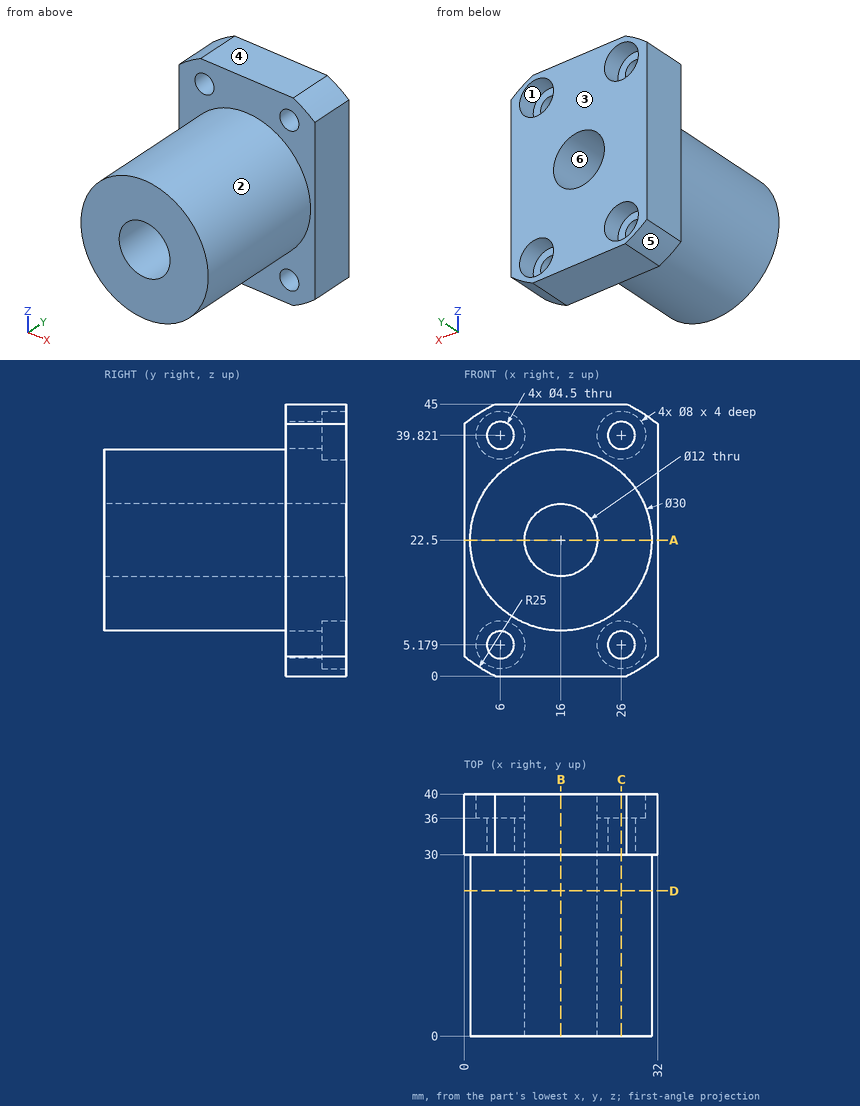
Study the drawing (mm; zero at the part's minimum x, y, z) and answer. A direction names the side the tool comes from. Coordinates: 2 decimals unless noted, no trailing zeros. Write each loop counter-clockwise with the first axis right and the second up, starting at its lowest first coordinate (ties: lowest second). Pieces come first, ordered by that corner, then holes. Notation, with made-up numbers: (29, 68) -> (49, 68) arc R16 cw to (49, 97) -> close; hole circle Ø1 at (61.5, 73.25). An arc over 180 degrees is marked (long way). Write each question's results on one line, items separated by ' | '. Start each with the question number.
1) A tool of negligible diameter and unlimited length cuts with its end or side. For the marked faces 1, 2 and 3, from which of +Z, -Z, +X, -X, +Y, -Y can it reach the whole face along a straight path? Write none if from no direction.
2) Straight lines are drawn through the part: probe 1 along Z at (x, y) = (6, 38.75); probe 2 along Z at (x, y) = (26, 32.8); probe 3 along Y at (x, z) = (25.5, 34.5). For each, find the intervals that lie inside material, in ascending order.
3) A cutting plane is placed at A-A (z = 22.5). Determine the outline of the cut face in (x, y).
4) A cutting plane is placed at D-D (y = 24). Determine the outline of the cut face in (x, z), then the cut area to 3 significant figures.
5) A cutting plane is placed at B-B (x = 16). Determine the outline of the cut face in (y, z).
6) Flat-ended cylindrical pins translate along their axes: pin 1 Ø4 at (x, z) = (7.5, 4.5) entering from +Y; pin 2 Ø5 at (x, z) = (6, 5.18) entering from -Y; pin 3 Ø2 at (y, z) = (11, 40) entering from -X; pin 4 Ø1 at (x, y) = (9.5, 27) entering from +Z. Find the tip coordinate at first contact, or state that the pin passes through.
7) For a pull along X with two mould halves and no side action, classify the marked faces 4, 5 and 6 as +X half, -X half, draft (parallel to the pull), parting line (faces both ways), or undercut.
8) A cutting plane is placed at C-C (x = 26). Determine the outline of the cut face in (y, z).
Values follow:
1) face 1: +Y | face 2: -Y | face 3: +Z, -Z, +X, -X, +Y
2) probe 1: 0 to 1.18, 9.18 to 35.82, 43.82 to 45 | probe 2: 0 to 2.93, 7.43 to 37.57, 42.07 to 45 | probe 3: 30 to 40
3) outline: (0, 30) -> (1, 30) -> (1, 0) -> (10, 0) -> (10, 40) -> (0, 40) -> close; (22, 0) -> (31, 0) -> (31, 30) -> (32, 30) -> (32, 40) -> (22, 40) -> close
4) outline: circle Ø30 at (16, 22.5); hole circle Ø12 at (16, 22.5) | area: 594 mm²
5) outline: (0, 7.5) -> (30, 7.5) -> (30, 0) -> (40, 0) -> (40, 16.5) -> (0, 16.5) -> close; (0, 28.5) -> (40, 28.5) -> (40, 45) -> (30, 45) -> (30, 37.5) -> (0, 37.5) -> close
6) pin 1: y = 36 | pin 2: y = 30 | pin 3: through | pin 4: z = 36.25
7) face 4: draft | face 5: -X half | face 6: undercut
8) outline: (0, 11.32) -> (30, 11.32) -> (30, 7.43) -> (36, 7.43) -> (36, 9.18) -> (40, 9.18) -> (40, 35.82) -> (36, 35.82) -> (36, 37.57) -> (30, 37.57) -> (30, 33.68) -> (0, 33.68) -> close; (30, 0) -> (40, 0) -> (40, 1.18) -> (36, 1.18) -> (36, 2.93) -> (30, 2.93) -> close; (30, 42.07) -> (36, 42.07) -> (36, 43.82) -> (40, 43.82) -> (40, 45) -> (30, 45) -> close
